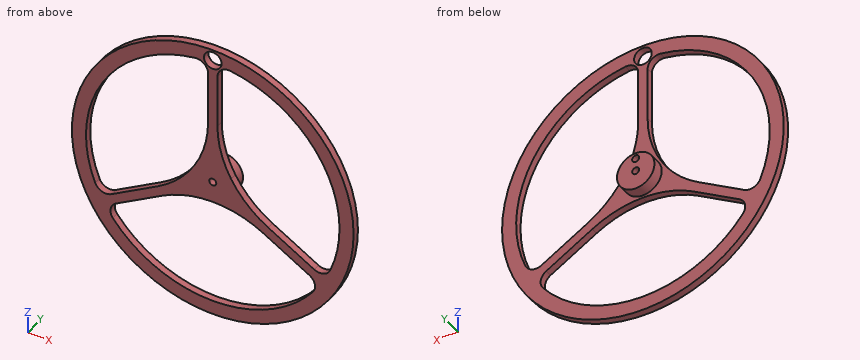
from build123d import *

# Parameters (mm, degrees)
SKETCH1_R           = 60
SKETCH1_R_2         = 54
SKETCH1_R_3         = 8
BOSS_EXTRUDE1_DEPTH = 3
SKETCH1_3_R         = 8
BOSS_EXTRUDE2_DEPTH = 5
CUT_EXTRUDE1_REACH  = 10
SKETCH2_R           = 1.5
CUT_EXTRUDE2_REACH  = 5
SKETCH3_R           = 3.75
SKETCH4_R           = 1.5
CUT_EXTRUDE3_DEPTH  = 5


with BuildPart() as part:
    # Sketch1 → Boss-Extrude1 (new body)
    with BuildSketch(Plane(origin=(0, 0, 0), x_dir=(1, 0, 0), z_dir=(0, 1, 0))):
        Circle(SKETCH1_R)
        Circle(SKETCH1_R_2, mode=Mode.SUBTRACT)
        with BuildLine():
            ThreePointArc((7.5, -53.47663041), (3.660460389, -52.338407931), (2.000000204, -48.694167705))
            Line((2.000000204, -48.694167705), (2.000000204, -26.12435489))
            ThreePointArc((2.000000204, -26.12435489), (3.473664254, -14.930765123), (7.794228634, -4.5))
            ThreePointArc((7.794228634, -4.5), (14.667254021, 4.457101073), (23.624355095, 11.33012646))
            Line((23.624355095, 11.33012646), (43.170386351, 22.615032868))
            ThreePointArc((43.170386351, 22.615032868), (47.156621056, 22.999152279), (50.062120444, 20.243124677))
            ThreePointArc((50.062120444, 20.243124677), (46.765371804, 27), (42.562120444, 33.233505733))
            ThreePointArc((42.562120444, 33.233505733), (43.496160667, 29.339255651), (41.170386147, 26.079134837))
            Line((41.170386147, 26.079134837), (21.62435489, 14.79422843))
            ThreePointArc((21.62435489, 14.79422843), (11.193589767, 10.47366405), (0, 9))
            ThreePointArc((0, 9), (-11.193589767, 10.47366405), (-21.62435489, 14.79422843))
            Line((-21.62435489, 14.79422843), (-41.170386147, 26.079134837))
            ThreePointArc((-41.170386147, 26.079134837), (-43.496160667, 29.339255651), (-42.562120444, 33.233505733))
            ThreePointArc((-42.562120444, 33.233505733), (-46.765371804, 27), (-50.062120444, 20.243124677))
            ThreePointArc((-50.062120444, 20.243124677), (-47.156621056, 22.999152279), (-43.170386351, 22.615032868))
            Line((-43.170386351, 22.615032868), (-23.624355095, 11.33012646))
            ThreePointArc((-23.624355095, 11.33012646), (-14.667254021, 4.457101073), (-7.794228634, -4.5))
            ThreePointArc((-7.794228634, -4.5), (-3.473664254, -14.930765123), (-2.000000204, -26.12435489))
            Line((-2.000000204, -26.12435489), (-2.000000204, -48.694167705))
            ThreePointArc((-2.000000204, -48.694167705), (-3.660460389, -52.338407931), (-7.5, -53.47663041))
            ThreePointArc((-7.5, -53.47663041), (0, -54), (7.5, -53.47663041))
        make_face()
        Circle(SKETCH1_R_3, mode=Mode.SUBTRACT)
        Circle(SKETCH1_R_3)
    extrude(amount=-BOSS_EXTRUDE1_DEPTH)

    # Sketch1_3 → Boss-Extrude2 (add)
    with BuildSketch(Plane(origin=(0, 0, 0), x_dir=(1, 0, 0), z_dir=(0, 1, 0))):
        Circle(SKETCH1_3_R)
    extrude(amount=BOSS_EXTRUDE2_DEPTH)

    # Sketch2 → Cut-Extrude1 (cut, up to next)
    with BuildSketch(Plane(origin=(0, 5, 0), x_dir=(1, 0, 0), z_dir=(0, 1, 0)), mode=Mode.PRIVATE) as cut_extrude1_sk1:
        Circle(SKETCH2_R)
    cut_extrude1_tool1 = extrude(cut_extrude1_sk1.sketch, amount=-CUT_EXTRUDE1_REACH, mode=Mode.PRIVATE) & part.part
    add(cut_extrude1_tool1.solids().sort_by_distance((0, 5, 0))[0], mode=Mode.SUBTRACT)

    # Sketch3 → Cut-Extrude2 (cut, up to next)
    with BuildSketch(Plane(origin=(0, 0, 0), x_dir=(1, 0, 0), z_dir=(0, 1, 0)), mode=Mode.PRIVATE) as cut_extrude2_sk1:
        with Locations((0, -55.25)):
            Circle(SKETCH3_R)
    cut_extrude2_tool1 = extrude(cut_extrude2_sk1.sketch, amount=-CUT_EXTRUDE2_REACH, mode=Mode.PRIVATE) & part.part
    add(cut_extrude2_tool1.solids().sort_by_distance((0, 0, 55.25))[0], mode=Mode.SUBTRACT)

    # Sketch4 → Cut-Extrude3 (cut)
    with BuildSketch(Plane(origin=(0, 5, 0), x_dir=(1, 0, 0), z_dir=(0, 1, 0))):
        with Locations((0, -5.5)):
            Circle(SKETCH4_R)
    extrude(amount=-CUT_EXTRUDE3_DEPTH, mode=Mode.SUBTRACT)


solid = part.part
For this review, take the finished solid that the model builds, in its own axes (mm). Round coordinates to 2 decimals unless told otherwise and drop trailing zeros. Loops run counter-clockwise (first coordinate to the right, second up) from the corner with the lowest first, then second, coordinate; pieces in that order, holes last. Notation, with made-up numbers: (78, -4.75) - (108, -4.75) arc R24 ccw to (108, 27.25) - close; hole circle Ø9 at (-32.75, -35.75). An arc over 180 degrees is marked (long way). One line per question, with ' | ' between items.
Q1. Take a section at A-A (x = 33.5). Give the boundary of the cut face in (y, z).
Taken from the geometry:
outline: (-3, -49.78) - (0, -49.78) - (0, -42.35) - (-3, -42.35) - close; (-3, -21.65) - (0, -21.65) - (0, -17.03) - (-3, -17.03) - close; (-3, 42.35) - (0, 42.35) - (0, 49.78) - (-3, 49.78) - close
Q2. For pin 1 (2.5 mm diameter, centred on y = -1.5, z = 42.5, fed in from -X); pin 2 (10 mm diameter, centred on x = 0, z = 55.25, fed in from +Y); pin 3 (1 mm diameter, centred on y = -1, z = 11.5, fed in from -X); pin 4 (2.5 mm diameter, centred on x = 0, z = 0, fed in from +Y), all flat-tipped, find the tip position at first contact; note any pin that passes through.
Taken from the geometry:
pin 1: stops at x = -43.57 | pin 2: stops at y = 0 | pin 3: stops at x = -58.98 | pin 4: passes through
Q3. For line 1 along Z through (x, y) = (-33.5, -2); line 2 along X through (y, z) = (-0.5, 34.5); line 3 along Z through (x, y) = (-43, -2.5), list the stretches that pass through material, from the lowest coordinate up. Write a range as [from, to].
Taken from the geometry:
line 1: z = [-49.78, -42.35], [-21.65, -17.03], [42.35, 49.78] | line 2: x = [-49.09, -41.54], [-2, 2], [41.54, 49.09] | line 3: z = [-41.84, -32.57], [-27.96, -22.52], [32.66, 41.84]
Q4. Take a section at C-C (x = 48). Give the boundary of the cut face in (y, z), and give its area (3 significant figures).
Taken from the geometry:
outline: (-3, -36) - (0, -36) - (0, -22.61) - (-3, -22.61) - close; (-3, 24.74) - (0, 24.74) - (0, 36) - (-3, 36) - close | area: 73.9 mm²
Q5. Take a section at B-B (z = 24.5). Give the boundary of the cut face in (x, y), and give its area (3 significant figures).
Taken from the geometry:
outline: (-54.77, -3) - (-48.12, -3) - (-48.12, 0) - (-54.77, 0) - close; (-2.03, -3) - (2.03, -3) - (2.03, 0) - (-2.03, 0) - close; (48.12, -3) - (54.77, -3) - (54.77, 0) - (48.12, 0) - close | area: 52.1 mm²
Q6. Take a section at D-D (z = 55.25). Give the boundary of the cut face in (x, y).
Taken from the geometry:
outline: (-23.4, -3) - (-3.75, -3) - (-3.75, 0) - (-23.4, 0) - close; (3.75, -3) - (23.4, -3) - (23.4, 0) - (3.75, 0) - close
